```python
from build123d import *

# Parameters (mm, degrees)
F2_T = -2.54


with BuildPart() as f1:
    # F0 (on Front) → F1 (revolve)
    with BuildSketch(Plane.XZ):
        Polygon((0, 0), (0, 66.7458474636), (-10.2124884725, 66.7458474636), (-10.2124884725, 58.6048029363), (-5.633150693, 58.6048029363), (-5.633150693, 36.7257446051), (-18.6927430332, 36.7257446051), (-18.6927430332, 0), align=None)
    revolve(axis=Axis((0, 0, 33.3729237318), (0, 0, -1)))

    # F2
    f2_openings = [f1.faces().sort_by_distance(p)[0] for p in [
        (0, 0, 66.745847),
    ]]
    offset(amount=F2_T, openings=f2_openings, kind=Kind.INTERSECTION)


solid = f1.part
```
Check sheet for the modelled part. Datum: model origin and axes. Units: mm. A direction names the side the tool comes from. Give positions to 0.01 mm unless a question says otherwise; leave off trailing zeros. Order: outer loops, then holes, each group sorted by start corner. A loop starts at its lowest first (then second) coordinate and runs counter-clockwise, first axis right, second up. Notation, with made-up numbers: (81, -18.75) -> (121, -18.75) arc R23 cw to (121, 12.25) -> close; hole circle Ø3 at (32.5, 56). An arc over 180 degrees is marked (long way). Use CSV: the item, a comma, the result in double quotes. Start each with the question number.
1) Go/stop test with flat-tipped pins: P1, Ø10, axis at x = 1.5, y = 3, coming from the -Z side; P2, Ø1.5, axis at x = 11, y = -7, coming from the +Z side; P3, Ø10, axis at y = 15, z = 30.5, coming from the +X side; P4, Ø1.5, axis at x = -11.5, z = 31, coming from the -Y side. Record where each tip stops, or that it passes through.
2) Material ranges on line 1 (Z direction, x = -1.5, y = 9.5); line 2 (Z direction, x = 0, y = 7.5); line 3 (Z direction, x = -9.5, y = -10.5), recorded low to high. Write a range as from..to.
3) Mould release check, pull along X, two halves, no side actions. Record for faces 4 (the face through (-4.4, -3.9, 36.726)), 5 (the face through (6.09, -4.67, 63.91)), 6 (the face through (13.78, 12.63, 18.11)): released by +X, released by -X, zero draft, split by the parting line, or undercut.
4) Sectioned sample at C-C, the plane y = 0. Record the boundary of the cut face in (x, z), plus the area to 3 significant figures.
5) Set-up check for faces 1 (the face through (1, 8, 66.746)), 2 (the face through (2.28, 2.09, 47.48)), 3 (the face through (-4.4, -4.4, 58.605)): record each of +Z, -Z, +X, -X, +Y, -Y from which the full face is reachable in a straight line by a thin tool's end or side.
6) Sectioned sample at A-A, the plane y = -6.5. Record the boundary of the cut face in (x, z).
7) Sectioned sample at B-B, the plane x = 4. Record the boundary of the cut face in (y, z), plus the area to 3 significant figures.
Recorded:
1,P1,"z = 0"
1,P2,"z = 36.73"
1,P3,"x = 15.79"
1,P4,"y = -15.29"
2,line 1,"0..2.54, 34.19..36.73, 58.6..66.75"
2,line 2,"0..2.54, 34.19..36.73, 58.6..61.14"
2,line 3,"0..2.54, 34.19..36.73"
3,face 4,"zero draft"
3,face 5,"undercut"
3,face 6,"split by the parting line"
4,outline,"(-18.69, 0) -> (18.69, 0) -> (18.69, 36.73) -> (5.63, 36.73) -> (5.63, 58.6) -> (10.21, 58.6) -> (10.21, 66.75) -> (7.67, 66.75) -> (7.67, 61.14) -> (3.09, 61.14) -> (3.09, 34.19) -> (16.15, 34.19) -> (16.15, 2.54) -> (-16.15, 2.54) -> (-16.15, 34.19) -> (-3.09, 34.19) -> (-3.09, 61.14) -> (-7.67, 61.14) -> (-7.67, 66.75) -> (-10.21, 66.75) -> (-10.21, 58.6) -> (-5.63, 58.6) -> (-5.63, 36.73) -> (-18.69, 36.73) -> close"
4,area,"511 mm2"
5,face 1,"+Z, +X, -X, +Y, -Y"
5,face 2,"+Z"
5,face 3,"none"
6,outline,"(-17.53, 0) -> (17.53, 0) -> (17.53, 36.73) -> (-17.53, 36.73) -> close; (-7.88, 58.6) -> (7.88, 58.6) -> (7.88, 66.75) -> (4.08, 66.75) -> (4.08, 61.14) -> (-4.08, 61.14) -> (-4.08, 66.75) -> (-7.88, 66.75) -> close; hole (-14.79, 2.54) -> (14.79, 2.54) -> (14.79, 34.19) -> (-14.79, 34.19) -> close"
7,outline,"(-18.26, 0) -> (18.26, 0) -> (18.26, 36.73) -> (3.97, 36.73) -> (3.97, 58.6) -> (9.4, 58.6) -> (9.4, 66.75) -> (6.55, 66.75) -> (6.55, 61.14) -> (-6.55, 61.14) -> (-6.55, 66.75) -> (-9.4, 66.75) -> (-9.4, 58.6) -> (-3.97, 58.6) -> (-3.97, 36.73) -> (-18.26, 36.73) -> close; hole (-15.65, 2.54) -> (15.65, 2.54) -> (15.65, 34.19) -> (-15.65, 34.19) -> close"
7,area,"604 mm2"
